Source: CAD feature listing. Evaluate the final solid. Frame: model axes, mm. Give positions to 0.01 mm unless a question says otherwise; leave off trailing zeros. Order: outer loops, then holes, each group sorted by start corner. A loop starts at its lowest first (then second) coordinate and runs counter-clockwise, first axis right, second up.
from build123d import *

# Parameters (mm, degrees)
SKETCH1_W              = 100
SKETCH1_H              = 65
BOSS_EXTRUDE1_DEPTH    = 6.35
M2_5_CLEARANCE_HOLE1_D = 2.9
SKETCH4_W              = 63
SKETCH4_H              = 29
CUT_EXTRUDE1_DEPTH     = 120.43752551
FILLET2_R              = 5
SKETCH5_W              = 12.5
SKETCH5_H              = 6.35
BOSS_EXTRUDE2_DEPTH    = 6.35
CUT_EXTRUDE2_DEPTH     = 120.43752551


with BuildPart() as part:
    # Sketch1 → Boss-Extrude1 (new body)
    with BuildSketch(Plane.XY):
        with Locations((50, 32.5)):
            Rectangle(SKETCH1_W, SKETCH1_H)
    extrude(amount=BOSS_EXTRUDE1_DEPTH)

    # M2.5 Clearance Hole1 (through all)
    with Locations(Plane.XY.offset(6.35)):
        with Locations((86, 57.3), (64, 57.3), (42, 57.3), (34.2, 51), (86, 22.7), (64, 22.7), (42, 22.7), (34.2, 29)):
            Hole(M2_5_CLEARANCE_HOLE1_D / 2)

    # Sketch4 → Cut-Extrude1 (cut, through all)
    with BuildSketch(Plane.XY.offset(6.35)):
        with Locations((68.5, 40)):
            Rectangle(SKETCH4_W, SKETCH4_H)
    extrude(amount=-CUT_EXTRUDE1_DEPTH, mode=Mode.SUBTRACT)

    # Fillet2
    fillet2_edges = [part.edges().sort_by_distance(p)[0] for p in [
        (0, 65, 3.175),
        (100, 65, 3.175),
        (100, 0, 3.175),
        (0, 0, 3.175),
    ]]
    fillet(fillet2_edges, radius=FILLET2_R)

    # Sketch5 → Boss-Extrude2 (add)
    with BuildSketch(Plane.XY.offset(6.35)):
        with Locations((69.75, -3.175)):
            Rectangle(SKETCH5_W, SKETCH5_H)
        with Locations((30.2758, -3.175)):
            Rectangle(SKETCH5_W, SKETCH5_H)
    extrude(amount=-BOSS_EXTRUDE2_DEPTH)

    # Sketch7 → Cut-Extrude2 (cut, through all)
    with BuildSketch(Plane(origin=(0, 0, 0), x_dir=(-1, 0, 0), z_dir=(0, 0, -1))):
        Polygon((-92.0271, 4.699), (-92.0271, 0), (-86.9471, 0), (-86.9471, 4.699), (-83.988, 4.699), (-83.988, 8.001), (-86.9471, 8.001), (-86.9471, 12.7), (-92.0271, 12.7), (-92.0271, 8.001), (-94.9862, 8.001), (-94.9862, 4.699), align=None)
        Polygon((-52.5529, 4.699), (-52.5529, 0), (-47.4729, 0), (-47.4729, 4.699), (-44.5138, 4.699), (-44.5138, 8.001), (-47.4729, 8.001), (-47.4729, 12.7), (-52.5529, 12.7), (-52.5529, 8.001), (-55.512, 8.001), (-55.512, 4.699), align=None)
        Polygon((-13.0787, 4.699), (-13.0787, 0), (-7.9987, 0), (-7.9987, 4.699), (-5.0396, 4.699), (-5.0396, 8.001), (-7.9987, 8.001), (-7.9987, 12.7), (-13.0787, 12.7), (-13.0787, 8.001), (-16.0378, 8.001), (-16.0378, 4.699), align=None)
    extrude(amount=-CUT_EXTRUDE2_DEPTH, mode=Mode.SUBTRACT)


solid = part.part
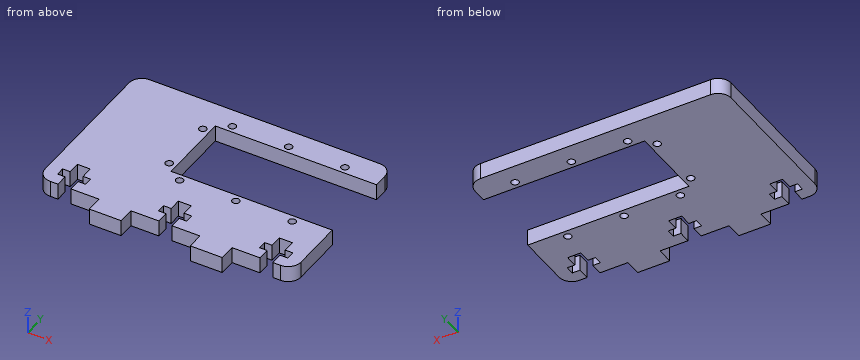
1) Section query B-B on x = 59.5. Output: boundary loops of the cut face in (y, z), and give its area (3 significant figures).
Checks:
outline: (0, 0) - (25.5, 0) - (25.5, 6.35) - (0, 6.35) - close; (54.5, 0) - (65, 0) - (65, 6.35) - (54.5, 6.35) - close
area: 229 mm2
2) Ray query, L1, parallel to Y at x = 42, z = 2; L2, parallel to Y at x = 45, z = 3.25; L3, parallel to X at y = 9, z = 1.5. Return the intervals inside material, ascending.
Checks:
L1: y = 0 to 21.25, 24.15 to 25.5, 54.5 to 55.85, 58.75 to 65
L2: y = 0 to 4.7, 8 to 25.5, 54.5 to 65
L3: x = 0 to 8, 13.08 to 47.47, 52.55 to 86.95, 92.03 to 100
3) First-contact query: pin 1 Ø0.9 at (x, z) = (6.5, 2.5) entering from -Y; pin 2 Ø1.9 at (y, z) = (-4, 3.5) entering from +X. Flat tips, straight axial feed; report the tip coordinate or a pass-through.
Checks:
pin 1: stops at y = 0
pin 2: stops at x = 76
4) Section query A-A on y = 51. Output: boundary loops of the cut face in (x, z), and give its area (3 significant figures).
Checks:
outline: (0, 0) - (32.75, 0) - (32.75, 6.35) - (0, 6.35) - close; (35.65, 0) - (37, 0) - (37, 6.35) - (35.65, 6.35) - close
area: 217 mm2
5) Section query D-D on z = 1. State how many separate pieces and enclosed holes the cut face has, and give its area (3 significant figures).
Checks:
separate pieces: 1
enclosed holes: 8
area: 4,510 mm2
6) Section query C-C on x = 42. Output: boundary loops of the cut face in (y, z).
Checks:
outline: (0, 0) - (21.25, 0) - (21.25, 6.35) - (0, 6.35) - close; (24.15, 0) - (25.5, 0) - (25.5, 6.35) - (24.15, 6.35) - close; (54.5, 0) - (55.85, 0) - (55.85, 6.35) - (54.5, 6.35) - close; (58.75, 0) - (65, 0) - (65, 6.35) - (58.75, 6.35) - close
